Print and shaded views of the part. All mm, measured from the part's lowest x, y and z. A direction names the side the tool comes from. Coordinates: 2 decimals unless noted, no trailing zeros. Order: outer loops, then holes, each group sorted by start corner. A loop starts at its lowest first (then second) coordinate and runs counter-clockwise, first axis right, second up. Notation, with made-up numbers: (4, 51) - (16, 51) arc R26 ccw to (16, 75) - close; hole circle Ø8 at (78, -4.75). An arc over 180 degrees is marked (long way). Write each question's results on one line, items separated by ' | '.
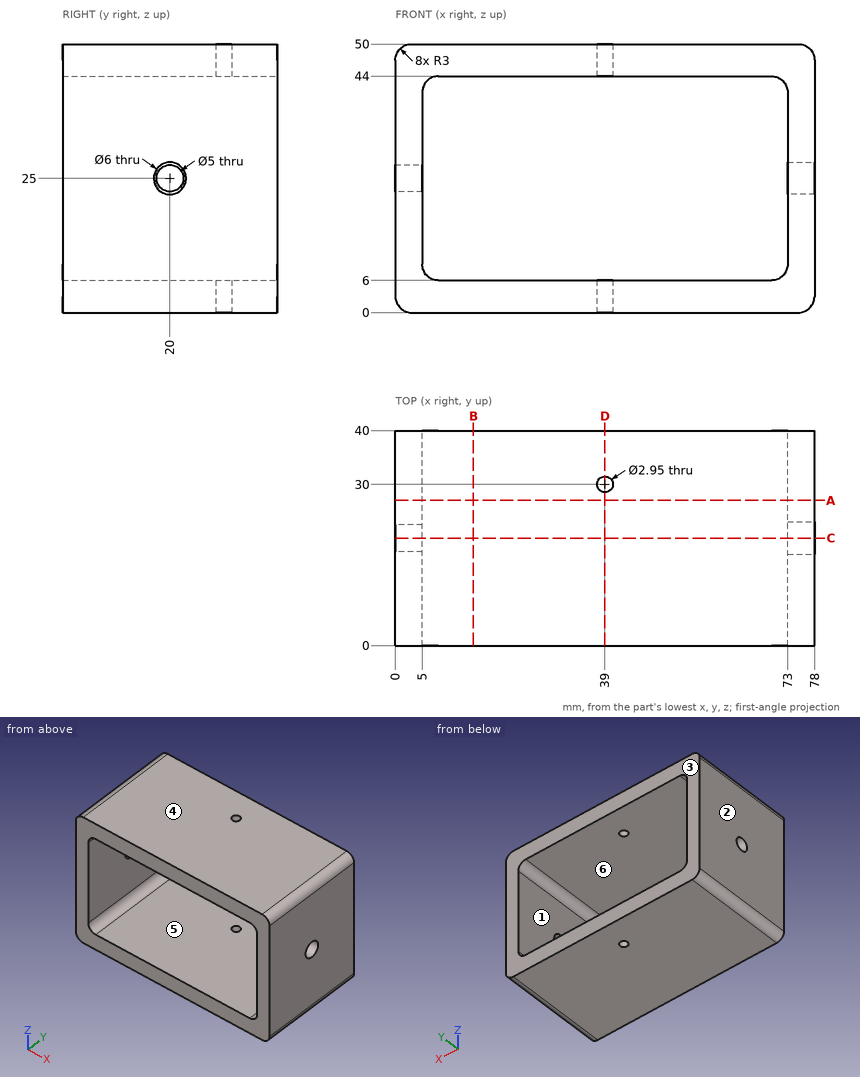
1. Band-saw the part on A-A on y = 27. Give the cut face in (x, z).
Solved:
outline: (0, 3) arc R3 ccw to (3, 0) - (75, 0) arc R3 ccw to (78, 3) - (78, 47) arc R3 ccw to (75, 50) - (3, 50) arc R3 ccw to (0, 47) - close; hole (5, 9) arc R3 ccw to (8, 6) - (70, 6) arc R3 ccw to (73, 9) - (73, 41) arc R3 ccw to (70, 44) - (8, 44) arc R3 ccw to (5, 41) - close
2. Two-plate mould, pull along Z, no slides. Class the marked faces 3, 4, 5 and 6: +Z half, -Z half, draft (parallel to the pull), parting line (faces both ways), or undercut.
Solved:
face 3: draft | face 4: +Z half | face 5: undercut | face 6: undercut
3. Tool access for the marked faces 1 and 2: list every direction of +Z, -Z, +X, -X, +Y, -Y with a clear straight run to the whole face (end or side of a thin tool).
Solved:
face 1: +Y, -Y | face 2: +Z, -Z, -X, +Y, -Y
4. Band-saw the part on D-D on x = 39. Give the cut face in (y, z) (3 decimals).
Solved:
outline: (0, 0) - (28.525, 0) - (28.525, 6) - (0, 6) - close; (0, 44) - (28.525, 44) - (28.525, 50) - (0, 50) - close; (31.475, 0) - (40, 0) - (40, 6) - (31.475, 6) - close; (31.475, 44) - (40, 44) - (40, 50) - (31.475, 50) - close
5. Probe line 1 (Y direction, x = 76.8, z = 25); line 2 (Z direction, x = 27, y = 24); line 3 (X direction, y = 7.5, z = 12). List the from-to ranges inside material, lowest first.
Solved:
line 1: y = 0 to 17, 23 to 40 | line 2: z = 0 to 6, 44 to 50 | line 3: x = 0 to 5, 73 to 78
6. Band-saw the part on C-C on y = 20. Give the cut face in (x, z), then the cut area to 3 significant figures.
Solved:
outline: (0, 3) arc R3 ccw to (3, 0) - (75, 0) arc R3 ccw to (78, 3) - (78, 22) - (73, 22) - (73, 9) arc R3 cw to (70, 6) - (8, 6) arc R3 cw to (5, 9) - (5, 22.5) - (0, 22.5) - close; (0, 27.5) - (5, 27.5) - (5, 41) arc R3 cw to (8, 44) - (70, 44) arc R3 cw to (73, 41) - (73, 28) - (78, 28) - (78, 47) arc R3 ccw to (75, 50) - (3, 50) arc R3 ccw to (0, 47) - close | area: 1,260 mm2
7. Band-saw the part on B-B on x = 14.5. Give the cut face in (y, z).
Solved:
outline: (0, 0) - (40, 0) - (40, 6) - (0, 6) - close; (0, 44) - (40, 44) - (40, 50) - (0, 50) - close
